Could you check a few things on this model? Use its own coordinates, in mm. Face numbers are marked on the shaded views. A direction names the side the tool comes from. Round coordinates to 2 decimals unless told otherwise and drop trailing zeros. Write each loop counter-clockwise with the first axis right and the second up, starting at its lowest first coordinate (ties: lowest second). Pieces come first, ordered by that corner, then holes.
```python
from build123d import *

# Parameters (mm, degrees)
CROQUIS1_R              = 9.5
SALIENTE_EXTRUIR1_DEPTH = 9
CROQUIS3_W              = 40
CROQUIS3_H              = 9
SALIENTE_EXTRUIR2_DEPTH = 12
CROQUIS4_R              = 2
CORTAR_EXTRUIR1_DEPTH   = 47.227697325
CROQUIS5_R              = 4
CORTAR_EXTRUIR2_DEPTH   = 4.5


with BuildPart() as part:
    # Croquis1 → Saliente-Extruir1 (new body)
    with BuildSketch(Plane.XY):
        with BuildLine():
            Line((-17, 22.5), (17, 22.5))
            ThreePointArc((17, 22.5), (19.121320344, 21.621320344), (20, 19.5))
            Line((20, 19.5), (20, -22.5))
            Line((20, -22.5), (-20, -22.5))
            Line((-20, -22.5), (-20, 19.5))
            ThreePointArc((-20, 19.5), (-19.121320344, 21.621320344), (-17, 22.5))
        make_face()
        with Locations((1, 7.5)):
            Circle(CROQUIS1_R, mode=Mode.SUBTRACT)
    extrude(amount=SALIENTE_EXTRUIR1_DEPTH)

    # Croquis3 → Saliente-Extruir2 (add)
    with BuildSketch(Plane.XY.offset(9)):
        with Locations((0, -18)):
            Rectangle(CROQUIS3_W, CROQUIS3_H)
    extrude(amount=SALIENTE_EXTRUIR2_DEPTH)

    # Croquis4 → Cortar-Extruir1 (cut, through all)
    with BuildSketch(Plane(origin=(0, -13.5, 0), x_dir=(1, 0, 0), z_dir=(0, 1, 0))):
        with Locations(Location((-10, -15, 0), (0, 0, 270))):
            Circle(CROQUIS4_R)
        with Locations(Location((10, -15, 0), (0, 0, 270))):
            Circle(CROQUIS4_R)
    extrude(amount=-CORTAR_EXTRUIR1_DEPTH, mode=Mode.SUBTRACT)

    # Croquis5 → Cortar-Extruir2 (cut)
    with BuildSketch(Plane(origin=(0, -13.5, 0), x_dir=(1, 0, 0), z_dir=(0, 1, 0))):
        with Locations(Location((-10, -15, 0), (0, 0, 270))):
            Circle(CROQUIS5_R)
        with Locations(Location((10, -15, 0), (0, 0, 270))):
            Circle(CROQUIS5_R)
    extrude(amount=-CORTAR_EXTRUIR2_DEPTH, mode=Mode.SUBTRACT)


solid = part.part
```
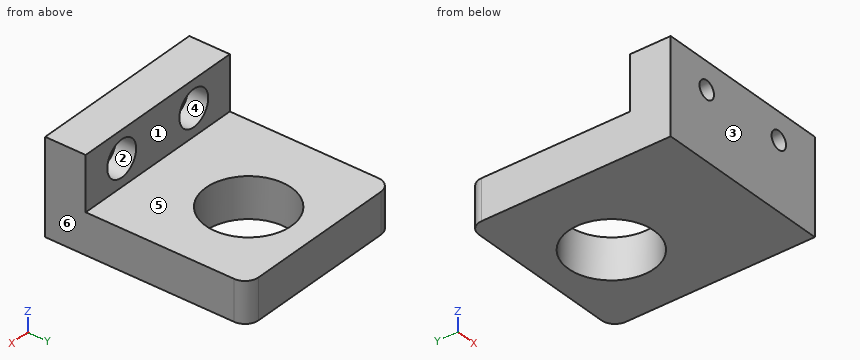
Q1. Imagine slicing it at B-B, the plane z = 15. Write out the boundary of the cut face in (x, y).
Q2. On a 3-axis mill with a long thin cutter (end or side, diameter ignored), from which of +Z, -Z, +X, -X, +Y, -Y can I reach the whole of each face in a straight line? I mean the marked faces 1, 2 and 3. Say none if no direction works.
Q3. I'm going to push flat-ended pins straight in: pin 1 Ø3 at (x, y) = (13, -18) entering from -Z; pin 2 Ø9 at (x, z) = (10, 15) entering from +Y; pin 3 Ø7 at (x, z) = (-10, 15) entering from +Y; pin 4 Ø18 at (x, y) = (-6, 2) entering from +Z. Where does each tip first touch, or does it pass through?
Q4. If I drill on L1, parallel to X at y = -19.8, z = 15; L2, parallel to Z at x = -9, y = -1; L3, parallel to Y at x = 5, z = 19, over which ranges is the centre line in solid material (lowest first)?
Q5. We'd pull the mould along Z, two halves only. Please class the marked faces 4, 5 and 6: pulls with the +Z half, pulls with the -Z half, needs draft (parallel to the pull), parting line crosses it, or undercut.
Q6. Imagine slicing it at A-A, the plane x = -10. Write out the boundary of the cut face in (y, z), then the cut area to 3 significant figures.
Q7. Imagine slicing it at D-D, the plane z = 2. Write out the boundary of the cut face in (x, y), then the cut area to 3 significant figures.
Q8. Imagine slicing it at C-C, the plane y = 7.5. Write out the boundary of the cut face in (x, z), then the cut area to 3 significant figures.
Results found:
1. outline: (-20, -22.5) - (-12, -22.5) - (-12, -18) - (-14, -18) - (-14, -13.5) - (-20, -13.5) - close; (-8, -22.5) - (8, -22.5) - (8, -18) - (6, -18) - (6, -13.5) - (-6, -13.5) - (-6, -18) - (-8, -18) - close; (12, -22.5) - (20, -22.5) - (20, -13.5) - (14, -13.5) - (14, -18) - (12, -18) - close
2. face 1: +Z, +X, -X, +Y
2. face 2: +Y
2. face 3: +Z, -Z, +X, -X, -Y
3. pin 1: stops at z = 0
3. pin 2: stops at y = -13.5
3. pin 3: stops at y = -18
3. pin 4: stops at z = 9
4. L1: x = -20 to -12, -8 to 8, 12 to 20
4. L2: z = 0 to 9
4. L3: y = -22.5 to -13.5
5. face 4: undercut
5. face 5: pulls with the +Z half
5. face 6: needs draft
6. outline: (-22.5, 0) - (22.5, 0) - (22.5, 9) - (-13.5, 9) - (-13.5, 11) - (-18, 11) - (-18, 13) - (-22.5, 13) - close; (-22.5, 17) - (-18, 17) - (-18, 19) - (-13.5, 19) - (-13.5, 21) - (-22.5, 21) - close
6. area: 459 mm2
7. outline: (-20, -22.5) - (20, -22.5) - (20, 19.5) arc R3 ccw to (17, 22.5) - (-17, 22.5) arc R3 ccw to (-20, 19.5) - close; hole circle Ø19 at (1, 7.5)
7. area: 1,510 mm2
8. outline: (-20, 0) - (-8.5, 0) - (-8.5, 9) - (-20, 9) - close; (10.5, 0) - (20, 0) - (20, 9) - (10.5, 9) - close
8. area: 189 mm2
